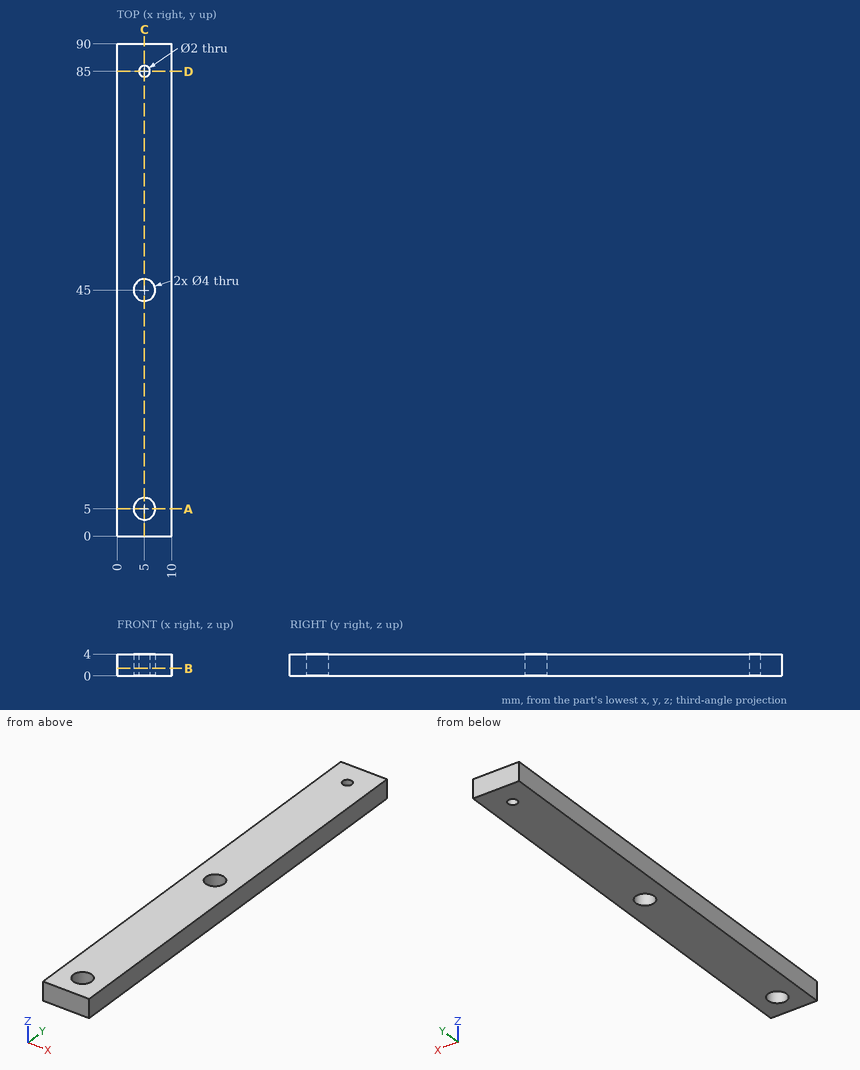
For this review, use the dimensioned drawing (mm, ordinates from the lowest corner) and the shaded views. Coordinates: 2 decimals unless noted, no trailing zeros. Loops run counter-clockwise (first coordinate to the right, second up) from the corner with the lowest first, then second, coordinate; pieces in that order, holes last. Notation, with made-up numbers: (-20.5, 4) -> (-5.5, 4) arc R22 cw to (-5.5, 16) -> close; hole circle Ø3 at (-30.75, -38). An arc over 180 degrees is marked (long way). Use a Markdown table: item, result. Add a question column.
Item 1: Wall thickness on L1, parallel to Y at x = 5, z = 1; L2, parallel to Y at x = 6.5, z = 0.2; L3, parallel to Y at x = 6.25, z = 1.25: over which ranges is each line inside the solid? List them lowest first. Write a range as from..to.
Item 2: We need section D-D, the plane y = 85. Write out the cut boundary in (x, z), and give its area (3 significant figures).
Item 3: Clearance check with a flat-ended pin moving along its axis: P1, Ø2.5, axis at x = 5, y = 5, coming from the -Z side. State where the tip first meets the part, or that it passes through.
Item 4: We need section C-C, the plane x = 5. Write out the cut boundary in (y, z).
Item 5: We need section A-A, the plane y = 5. Write out the cut boundary in (x, z).
Item 6: We need section B-B, the plane z = 1.4. Write out the cut boundary in (x, y), and give its area (3 significant figures).
Numbers:
| question | item | result |
|---|---|---|
| 1 | L1 | y = 0..3, 7..43, 47..84, 86..90 |
| 1 | L2 | y = 0..3.68, 6.32..43.68, 46.32..90 |
| 1 | L3 | y = 0..3.44, 6.56..43.44, 46.56..90 |
| 2 | outline | (0, 0) -> (4, 0) -> (4, 4) -> (0, 4) -> close; (6, 0) -> (10, 0) -> (10, 4) -> (6, 4) -> close |
| 2 | area | 32.0 mm^2 |
| 3 | P1 | passes through |
| 4 | outline | (0, 0) -> (3, 0) -> (3, 4) -> (0, 4) -> close; (7, 0) -> (43, 0) -> (43, 4) -> (7, 4) -> close; (47, 0) -> (84, 0) -> (84, 4) -> (47, 4) -> close; (86, 0) -> (90, 0) -> (90, 4) -> (86, 4) -> close |
| 5 | outline | (0, 0) -> (3, 0) -> (3, 4) -> (0, 4) -> close; (7, 0) -> (10, 0) -> (10, 4) -> (7, 4) -> close |
| 6 | outline | (0, 0) -> (10, 0) -> (10, 90) -> (0, 90) -> close; hole circle Ø4 at (5, 5); hole circle Ø4 at (5, 45); hole circle Ø2 at (5, 85) |
| 6 | area | 872 mm^2 |
